Source: CAD feature listing. Evaluate the final solid. Frame: model axes, mm. A direction names the side the tool comes from. Give positions to 0.01 mm unless a question says otherwise; leave off trailing zeros. Loops run counter-clockwise (first coordinate to the right, second up) from the corner with the lowest first, then second, coordinate; pieces in that order, holes last. Notation, with made-up numbers: M -16.5,6 L 25.5,6 A7 ccw 25.5,17 Z; hole C 5,80 d6. An arc over 180 degrees is marked long. Answer in a Markdown table with one row per item.
```python
from build123d import *

# Parameters (mm, degrees)
BOSS_EXTRUDE1_DEPTH                = 26
CUT_EXTRUDE1_DEPTH                 = 14
CUT_EXTRUDE2_DEPTH                 = 47
CUT_EXTRUDE3_DEPTH                 = 2
SKETCH5_R                          = 2
CUT_EXTRUDE4_DEPTH                 = 178.493661859
MIRROR2_COPY_1_SKETCH_R            = 2
MIRROR2_COPY_1_DEPTH               = 178.493661859
CUT_EXTRUDE5_DEPTH                 = 12
CUT_EXTRUDE6_START                 = -2
CUT_EXTRUDE6_DEPTH                 = 2
F_3_0_3_DIAMETER_HOLE3_D           = 3
M3_CLEARANCE_HOLE2_D               = 3.4
M3_CLEARANCE_HOLE2_DEPTH           = 20
M3_CLEARANCE_HOLE2_ON_FACE_2_D     = 3.4
M3_CLEARANCE_HOLE2_ON_FACE_2_DEPTH = 20
M3_CLEARANCE_HOLE2_ON_FACE_3_D     = 3.4
M3_CLEARANCE_HOLE2_ON_FACE_3_DEPTH = 20
M3_CLEARANCE_HOLE2_ON_FACE_4_D     = 3.4
M3_CLEARANCE_HOLE2_ON_FACE_4_DEPTH = 20
CUT_EXTRUDE7_DEPTH                 = 10
CUT_EXTRUDE8_DEPTH                 = 10
M3X0_5_TAPPED_HOLE1_D              = 2.5
M3X0_5_TAPPED_HOLE1_DEPTH          = 7.5
M3X0_5_TAPPED_HOLE1_TIP            = 0.751075774


with BuildPart() as part:
    # Sketch1 → Boss-Extrude1 (new, symmetric)
    with BuildSketch(Plane(origin=(0, 0, 0), x_dir=(1, 0, 0), z_dir=(0, 1, 0))):
        with BuildLine():
            Line((-100, 120), (-120, 120))
            Line((-120, 120), (-120, 100))
            Line((-120, 100), (-110, 100))
            ThreePointArc((-110, 100), (-102.928932188, 97.071067812), (-100, 90))
            Line((-100, 90), (-100, 0))
            Line((-100, 0), (-100, -90))
            ThreePointArc((-100, -90), (-102.928932188, -97.071067812), (-110, -100))
            Line((-110, -100), (-120, -100))
            Line((-120, -100), (-120, -120))
            Line((-120, -120), (-100, -120))
            Line((-100, -120), (-100, -110))
            ThreePointArc((-100, -110), (-97.071067812, -102.928932188), (-90, -100))
            Line((-90, -100), (0, -100))
            Line((0, -100), (90, -100))
            ThreePointArc((90, -100), (97.071067812, -102.928932188), (100, -110))
            Line((100, -110), (100, -120))
            Line((100, -120), (120, -120))
            Line((120, -120), (120, -100))
            Line((120, -100), (110, -100))
            ThreePointArc((110, -100), (102.928932188, -97.071067812), (100, -90))
            Line((100, -90), (100, 0))
            Line((100, 0), (100, 90))
            ThreePointArc((100, 90), (102.928932188, 97.071067812), (110, 100))
            Line((110, 100), (120, 100))
            Line((120, 100), (120, 120))
            Line((120, 120), (100, 120))
            Line((100, 120), (100, 110))
            ThreePointArc((100, 110), (97.071067812, 102.928932188), (90, 100))
            Line((90, 100), (0, 100))
            Line((0, 100), (-90, 100))
            ThreePointArc((-90, 100), (-97.071067812, 102.928932188), (-100, 110))
            Line((-100, 110), (-100, 120))
        make_face()
    extrude(amount=BOSS_EXTRUDE1_DEPTH, both=True)

    # Sketch2 → Cut-Extrude1 (cut)
    with BuildSketch(Plane.XZ):
        Polygon((-120, -100.707106781), (-100.707106781, -120), (-120, -120), align=None)
        Polygon((-100.707106781, 120), (-120, 120), (-120, 100.707106781), align=None)
        Polygon((120, 100.707106781), (120, 120), (100.707106781, 120), align=None)
        Polygon((100.707106781, -120), (120, -120), (120, -100.707106781), align=None)
    extrude(amount=-CUT_EXTRUDE1_DEPTH, mode=Mode.SUBTRACT)

    # Sketch3 → Cut-Extrude2 (cut)
    with BuildSketch(Plane(origin=(0, 26, 0), x_dir=(1, 0, 0), z_dir=(0, 1, 0))):
        with BuildLine():
            Line((-88, 98), (88, 98))
            ThreePointArc((88, 98), (95.071067812, 95.071067812), (98, 88))
            Line((98, 88), (98, -88))
            ThreePointArc((98, -88), (95.071067812, -95.071067812), (88, -98))
            Line((88, -98), (-88, -98))
            ThreePointArc((-88, -98), (-95.071067812, -95.071067812), (-98, -88))
            Line((-98, -88), (-98, 88))
            ThreePointArc((-98, 88), (-95.071067812, 95.071067812), (-88, 98))
        make_face()
    extrude(amount=-CUT_EXTRUDE2_DEPTH, mode=Mode.SUBTRACT)

    # Sketch4 → Cut-Extrude3 (cut)
    with BuildSketch(Plane(origin=(0, -21, 0), x_dir=(1, 0, 0), z_dir=(0, 1, 0))):
        with BuildLine():
            Line((-88, -96), (88, -96))
            ThreePointArc((88, -96), (93.656854249, -93.656854249), (96, -88))
            Line((96, -88), (96, 88))
            ThreePointArc((96, 88), (93.656854249, 93.656854249), (88, 96))
            Line((88, 96), (-88, 96))
            ThreePointArc((-88, 96), (-93.656854249, 93.656854249), (-96, 88))
            Line((-96, 88), (-96, -88))
            ThreePointArc((-96, -88), (-93.656854249, -93.656854249), (-88, -96))
        make_face()
    extrude(amount=-CUT_EXTRUDE3_DEPTH, mode=Mode.SUBTRACT)

    # Sketch5 → Cut-Extrude4 (cut, through all)
    with BuildSketch(Plane(origin=(0, 26, 0), x_dir=(1, 0, 0), z_dir=(0, 1, 0))):
        with Locations(Location((-112, 112, 0), (0, 0, 270))):
            Circle(SKETCH5_R)
    cut_extrude4 = extrude(amount=-CUT_EXTRUDE4_DEPTH, mode=Mode.SUBTRACT)

    # Mirror1: Cut-Extrude4 across plane
    add(cut_extrude4.mirror(Plane(origin=(0, 0, 0), x_dir=(0, 0, 1), z_dir=(1, 0, 0))), mode=Mode.SUBTRACT)

    # Mirror2: Cut-Extrude4 across plane
    add(cut_extrude4.mirror(Plane.XY), mode=Mode.SUBTRACT)

    # Mirror2 copy 1 sketch → Mirror2 copy 1 (cut, through all)
    with BuildSketch(Plane(origin=(0, 26, 0), x_dir=(-1, 0, 0), z_dir=(0, 1, 0))):
        with Locations(Location((-112, 112, 0), (0, 0, 270))):
            Circle(MIRROR2_COPY_1_SKETCH_R)
    extrude(amount=-MIRROR2_COPY_1_DEPTH, mode=Mode.SUBTRACT)

    # Sketch2<3> → Cut-Extrude5 (cut)
    with BuildSketch(Plane.XZ):
        Polygon((-120, -100.707106781), (-100.707106781, -120), (-120, -120), align=None)
        Polygon((-100.707106781, 120), (-120, 120), (-120, 100.707106781), align=None)
        Polygon((120, 100.707106781), (120, 120), (100.707106781, 120), align=None)
        Polygon((100.707106781, -120), (120, -120), (120, -100.707106781), align=None)
    extrude(amount=CUT_EXTRUDE5_DEPTH, mode=Mode.SUBTRACT)

    # Sketch14 → Cut-Extrude6 (cut)
    with BuildSketch(Plane.XZ.offset(26).offset(CUT_EXTRUDE6_START)):
        with BuildLine():
            Line((-90, -100), (90, -100))
            ThreePointArc((90, -100), (97.071067812, -102.928932188), (100, -110))
            Line((100, -110), (100, -120))
            Line((100, -120), (120, -120))
            Line((120, -120), (120, -100))
            Line((120, -100), (110, -100))
            ThreePointArc((110, -100), (102.928932188, -97.071067812), (100, -90))
            Line((100, -90), (100, 90))
            ThreePointArc((100, 90), (102.928932188, 97.071067812), (110, 100))
            Line((110, 100), (120, 100))
            Line((120, 100), (120, 120))
            Line((120, 120), (100, 120))
            Line((100, 120), (100, 110))
            ThreePointArc((100, 110), (97.071067812, 102.928932188), (90, 100))
            Line((90, 100), (-90, 100))
            ThreePointArc((-90, 100), (-97.071067812, 102.928932188), (-100, 110))
            Line((-100, 110), (-100, 120))
            Line((-100, 120), (-120, 120))
            Line((-120, 120), (-120, 100))
            Line((-120, 100), (-110, 100))
            ThreePointArc((-110, 100), (-102.928932188, 97.071067812), (-100, 90))
            Line((-100, 90), (-100, -90))
            ThreePointArc((-100, -90), (-102.928932188, -97.071067812), (-110, -100))
            Line((-110, -100), (-120, -100))
            Line((-120, -100), (-120, -120))
            Line((-120, -120), (-100, -120))
            Line((-100, -120), (-100, -110))
            ThreePointArc((-100, -110), (-97.071067812, -102.928932188), (-90, -100))
        make_face()
        with BuildLine():
            Line((-88, 98), (88, 98))
            ThreePointArc((88, 98), (95.071067812, 95.071067812), (98, 88))
            Line((98, 88), (98, -88))
            ThreePointArc((98, -88), (95.071067812, -95.071067812), (88, -98))
            Line((88, -98), (-88, -98))
            ThreePointArc((-88, -98), (-95.071067812, -95.071067812), (-98, -88))
            Line((-98, -88), (-98, 88))
            ThreePointArc((-98, 88), (-95.071067812, 95.071067812), (-88, 98))
        make_face(mode=Mode.SUBTRACT)
    extrude(amount=CUT_EXTRUDE6_DEPTH, mode=Mode.SUBTRACT)

    # Ø3.0 (3) Diameter Hole3 (through all)
    with Locations(Plane(origin=(0, -23, 0), x_dir=(1, 0, 0), z_dir=(0, 1, 0))):
        with Locations((-90, 79.8), (-50, 79.8), (-50, 26.6), (-90, 26.6), (-90, -26.6), (-50, -26.6), (-50, -79.8), (-90, -79.8), (-35.25, -60), (0, -60), (35.25, -60), (50, -79.8), (90, -79.8), (90, -26.6), (50, -26.6), (50, 26.6), (90, 26.6), (90, 79.8), (50, 79.8)):
            Hole(F_3_0_3_DIAMETER_HOLE3_D / 2)

    # M3 Clearance Hole2
    with Locations(Plane(origin=(-116, 20, 120), x_dir=(1, 0, 0), z_dir=(0, 0, 1))):
        with Locations((0, 0), (232, -38)):
            Hole(M3_CLEARANCE_HOLE2_D / 2, depth=M3_CLEARANCE_HOLE2_DEPTH)

    # M3 Clearance Hole2 on face 2
    with Locations(Plane(origin=(120, 20, 116), x_dir=(0, 0, 1), z_dir=(1, 0, 0))):
        with Locations((0, 0), (-232, 38)):
            Hole(M3_CLEARANCE_HOLE2_ON_FACE_2_D / 2, depth=M3_CLEARANCE_HOLE2_ON_FACE_2_DEPTH)

    # M3 Clearance Hole2 on face 3
    with Locations(Plane(origin=(116, 20, -120), x_dir=(-1, 0, 0), z_dir=(0, 0, -1))):
        with Locations((0, 0), (232, -38)):
            Hole(M3_CLEARANCE_HOLE2_ON_FACE_3_D / 2, depth=M3_CLEARANCE_HOLE2_ON_FACE_3_DEPTH)

    # M3 Clearance Hole2 on face 4
    with Locations(Plane(origin=(-120, 20, -116), x_dir=(0, 0, -1), z_dir=(-1, 0, 0))):
        with Locations((0, 0), (-232, 38)):
            Hole(M3_CLEARANCE_HOLE2_ON_FACE_4_D / 2, depth=M3_CLEARANCE_HOLE2_ON_FACE_4_DEPTH)

    # Sketch26 → Cut-Extrude7 (cut)
    with BuildSketch(Plane.XY.offset(100)):
        with BuildLine():
            Line((-26.935894027, 10.57), (-13.064105973, 10.57))
            ThreePointArc((-13.064105973, 10.57), (-10.497857088, 9.373338492), (-9.765, 6.638278605))
            Line((-9.765, 6.638278605), (-10.593736809, 1.938278605))
            ThreePointArc((-10.593736809, 1.938278605), (-11.739504289, -0.046248884), (-13.892842782, -0.83))
            Line((-13.892842782, -0.83), (-26.107157218, -0.83))
            ThreePointArc((-26.107157218, -0.83), (-28.260495711, -0.046248884), (-29.406263191, 1.938278605))
            Line((-29.406263191, 1.938278605), (-30.235, 6.638278605))
            ThreePointArc((-30.235, 6.638278605), (-29.502142912, 9.373338492), (-26.935894027, 10.57))
        make_face()
    extrude(amount=-CUT_EXTRUDE7_DEPTH, mode=Mode.SUBTRACT)

    # Sketch27 → Cut-Extrude8 (cut)
    with BuildSketch(Plane.XY.offset(100)):
        with BuildLine():
            Line((13.064105973, 10.57), (26.935894027, 10.57))
            ThreePointArc((26.935894027, 10.57), (29.502142912, 9.373338492), (30.235, 6.638278605))
            Line((30.235, 6.638278605), (29.406263191, 1.938278605))
            ThreePointArc((29.406263191, 1.938278605), (28.260495711, -0.046248884), (26.107157218, -0.83))
            Line((26.107157218, -0.83), (13.892842782, -0.83))
            ThreePointArc((13.892842782, -0.83), (11.739504289, -0.046248884), (10.593736809, 1.938278605))
            Line((10.593736809, 1.938278605), (9.765, 6.638278605))
            ThreePointArc((9.765, 6.638278605), (10.497857088, 9.373338492), (13.064105973, 10.57))
        make_face()
    extrude(amount=-CUT_EXTRUDE8_DEPTH, mode=Mode.SUBTRACT)

    # M3x0.5 Tapped Hole1
    with Locations(Plane.XY.offset(100)):
        with Locations((-32.495, 4.86), (-7.505, 4.86), (7.505, 4.86), (32.495, 4.86)):
            Hole(M3X0_5_TAPPED_HOLE1_D / 2, depth=M3X0_5_TAPPED_HOLE1_DEPTH)
            with Locations((0, 0, -(M3X0_5_TAPPED_HOLE1_DEPTH + M3X0_5_TAPPED_HOLE1_TIP / 2))):  # 118° drill point
                Cone(0, M3X0_5_TAPPED_HOLE1_D / 2, M3X0_5_TAPPED_HOLE1_TIP, mode=Mode.SUBTRACT)


solid = part.part
```
1) Pull-direction query (X, two-part tool) for faces 1 (the flat face through (-113, 14, 115)), 2 (the flat face through (-98, 3, 1)), 3 (the cylindrical face through (-94.99, -24.99, -95.15)); classes: released by +X, released by -X, zero draft, split by the parting line, or undercut.
Reply:
| item | result |
|---|---|
| face 1 | zero draft |
| face 2 | undercut |
| face 3 | released by -X |
2) Section A-A, the plane z = -52. Return loops of the section in (x, y).
Reply:
| item | result |
|---|---|
| outline | M -100,-24 L -98,-24 L -98,-26 L 98,-26 L 98,-24 L 100,-24 L 100,26 L 98,26 L 98,-21 L 96,-21 L 96,-23 L -96,-23 L -96,-21 L -98,-21 L -98,26 L -100,26 Z |
3) Pin query (flat end, axial travel): pin 1 Ø3.5 at (x, z) = (-112, 112) entering from +Y; pin 2 Ø10 at (x, z) = (-95.5, -71.5) entering from +Y; pin 3 Ø5 at (x, z) = (-112, 112) entering from -Y; pin 4 Ø2 at (x, y) = (79, -5) entering from +Z. Return the tip coordinate at first contact, or that it passes through.
Reply:
| item | result |
|---|---|
| pin 1 | passes through |
| pin 2 | stops at y = 26 |
| pin 3 | stops at y = -24 |
| pin 4 | stops at z = 100 |
4) Set-up query: faces 4 (the cylindrical face through (-95.15, -24.99, 94.99)), 5 (the cylindrical face through (103.01, 1.35, 97.15)), 6 (the flat face through (115, 14, -115)), 7 (the cylindrical face through (96.99, 1.35, 102.85)). Return all of +Z, -Z, +X, -X, +Y, -Y with unobstructed straight access to the full face (end or side cutting, diameter ignored); none if empty.
Reply:
| item | result |
|---|---|
| face 4 | +Z, -X, -Y |
| face 5 | +X, +Y, -Y |
| face 6 | -Z, +X |
| face 7 | +Z, +Y, -Y |
5) Material intervals for L1, parallel to Y at x = 116, z = -110; L2, parallel to Z at x = -50, y = -24.1; L3, parallel to X at y = -3, z = 27, sorted ascending.
Reply:
| item | result |
|---|---|
| L1 | y = -24 to -12, 14 to 18.3, 21.7 to 26 |
| L2 | z = -98 to -81.3, -78.3 to -28.1, -25.1 to 25.1, 28.1 to 78.3, 81.3 to 98 |
| L3 | x = -100 to -98, 98 to 100 |
